Part model, mm, in its own coordinate system. Coordinates: 2 decimals unless noted, no trailing zeros. Loops run counter-clockwise (first coordinate to the right, second up) from the corner with the lowest first, then second, coordinate; pieces in that order, holes last. Notation, with made-up numbers: (-3, -10.75) -> (44, -10.75) arc R9 ccw to (44, 2.25) -> close; hole circle Ø11 at (88, 88). An arc over 180 degrees is marked (long way). Use one line per item in the form item = value. Start each with the question number.
(1) Drill centre lines: L1, parallel to X at y = 5.75, z = 9; L2, parallel to X at y = 13.5, z = 8; L3, parallel to Y at x = 9, z = 22.5. Where is each one in solid material? Low to high. Write a range as [from, to].
(2) Band-saw the part on A-A on z = 23.5. Give the cut face in (x, y).
(3) Pin check, flat tips, straight feed: P1, Ø1.5, axis at y = 4.5, z = 3.5, coming from the +X side; P2, Ø1, axis at y = 5, z = 21.5, coming from the +X side; P3, Ø2, axis at y = 2, z = -3, coming from the +X side. Stop position of each tip, or through.
```python
from build123d import *

# Parameters (mm, degrees)
F0_W         = 15.478125
F0_H         = 15.478125
F1_DEPTH     = 6.35
F2_DEPTH     = 25.4
F2_TAPER     = 10
F3_T1_DEPTH  = 51.3009034407
F3_T3_DEPTH  = 51.3009034407
F3_T5_DEPTH  = 51.3009034407
F3_T7_DEPTH  = 51.3009034407
F3_T9_DEPTH  = 44.45
F3_T11_DEPTH = 0.1267751904
F3_T13_DEPTH = 0.1267751904
F3_S17_W     = 14.1899336178
F3_S17_H     = 14.1899336178
F3_T18_DEPTH = 7.0949668089
F3_S29_W     = 14.1899336177
F3_S29_H     = 14.1899336178
F3_T30_DEPTH = 7.0949668089
F3_S41_W     = 14.1899336177
F3_S41_H     = 14.1899336178
F3_T42_DEPTH = 7.0949668089
F3_S53_W     = 14.1899336178
F3_S53_H     = 14.1899336178
F3_T54_DEPTH = 7.0949668089


# Not quite as in the source:
# - a fillet or chamfer that OpenCascade refuses, or shapes differently, is made with other operations: its cross-section is extruded or revolved along the edge and cut away or added


with BuildPart() as f1:
    # F0 (on Top) → F1 (new body)
    with BuildSketch(Plane.XY):
        with Locations((7.7390625, 7.7390625)):
            Rectangle(F0_W, F0_H)
    extrude(amount=-F1_DEPTH)

    # F0 (on Top) → F2 (join)
    with BuildSketch(Plane.XY):
        with Locations((7.7390625, 7.7390625)):
            Rectangle(F0_W, F0_H)
    extrude(amount=F2_DEPTH, taper=F2_TAPER)

    # F3: fillet of radius 3.81 on 10 edges, made by hand

    # F3_s2 → F3_t1 (cut)
    with BuildSketch(Plane(origin=(5.649698691, 5.649698691, -32.0410334724), x_dir=(0.7071067812, -0.7071067812, 0), z_dir=(-0.1710878697, -0.1710878697, 0.9702875252))):
        with BuildLine():
            ThreePointArc((-2.6531477556, 18.6646706441), (0, 19.7402772951), (2.6531477556, 18.6646706441))
            Line((2.6531477556, 18.6646706441), (0, 21.238986814))
            Line((0, 21.238986814), (-2.6531477556, 18.6646706441))
        make_face()
    extrude(amount=F3_T1_DEPTH, mode=Mode.SUBTRACT)

    # F3_s4 → F3_t3 (cut)
    with BuildSketch(Plane(origin=(-5.1966375782, 5.1966375782, -29.4715962203), x_dir=(0.7071067812, 0.7071067812, 0), z_dir=(0.1710878697, -0.1710878697, 0.9702875252))):
        with BuildLine():
            ThreePointArc((8.2915393919, 8.0451772371), (10.9446871476, 9.1207838881), (13.5978349032, 8.0451772371))
            Line((13.5978349032, 8.0451772371), (10.9446871476, 10.619493407))
            Line((10.9446871476, 10.619493407), (8.2915393919, 8.0451772371))
        make_face()
    extrude(amount=F3_T3_DEPTH, mode=Mode.SUBTRACT)

    # F3_s6 → F3_t5 (cut)
    with BuildSketch(Plane(origin=(5.1966375782, -5.1966375782, -29.4715962203), x_dir=(-0.7071067812, -0.7071067812, 0), z_dir=(-0.1710878697, 0.1710878697, 0.9702875252))):
        with BuildLine():
            ThreePointArc((-8.2915393919, 8.0451772371), (-10.9446871476, 9.1207838881), (-13.5978349032, 8.0451772371))
            Line((-13.5978349032, 8.0451772371), (-10.9446871476, 10.619493407))
            Line((-10.9446871476, 10.619493407), (-8.2915393919, 8.0451772371))
        make_face()
    extrude(amount=F3_T5_DEPTH, mode=Mode.SUBTRACT)

    # F3_s8 → F3_t7 (cut)
    with BuildSketch(Plane(origin=(-4.7435764654, -4.7435764654, -26.9021589682), x_dir=(-0.7071067812, 0.7071067812, 0), z_dir=(0.1710878697, 0.1710878697, 0.9702875252))):
        with BuildLine():
            ThreePointArc((2.6531477556, -2.5743161699), (0, -1.4987095189), (-2.6531477556, -2.5743161699))
            Line((-2.6531477556, -2.5743161699), (0, 0))
            Line((0, 0), (2.6531477556, -2.5743161699))
        make_face()
    extrude(amount=F3_T7_DEPTH, mode=Mode.SUBTRACT)

    # F3_s10 → F3_t9 (cut)
    with BuildSketch(Plane.XY.offset(-15.875)):
        with BuildLine():
            ThreePointArc((0, 3.81), (1.1159231637, 1.1159231637), (3.81, 0))
            Line((3.81, 0), (0, 0))
            Line((0, 0), (0, 3.81))
        make_face()
        with BuildLine():
            ThreePointArc((11.668125, 0), (14.3622018363, 1.1159231637), (15.478125, 3.81))
            Line((15.478125, 3.81), (15.478125, 0))
            Line((15.478125, 0), (11.668125, 0))
        make_face()
    extrude(amount=F3_T9_DEPTH, mode=Mode.SUBTRACT)

    # F3_s12 → F3_t11 (cut)
    with BuildSketch(Plane.XZ.offset(-7.8024500952)):
        with BuildLine():
            ThreePointArc((7.8024500952, 25.4), (10.2514708881, 24.5086293283), (11.5545676342, 22.2515995569))
            Line((11.5545676342, 22.2515995569), (10.99941969, 25.4))
            Line((10.99941969, 25.4), (7.8024500952, 25.4))
        make_face()
        with BuildLine():
            ThreePointArc((3.9235573658, 22.2515995569), (5.2266541119, 24.5086293283), (7.6756749048, 25.4))
            Line((7.6756749048, 25.4), (4.47870531, 25.4))
            Line((4.47870531, 25.4), (3.9235573658, 22.2515995569))
        make_face()
    extrude(amount=F3_T11_DEPTH, mode=Mode.SUBTRACT)

    # F3_s14 → F3_t13 (cut)
    with BuildSketch(Plane.YZ.offset(7.6756749048)):
        with BuildLine():
            ThreePointArc((3.9235573658, 22.2515995569), (5.2266541119, 24.5086293283), (7.6756749048, 25.4))
            Line((7.6756749048, 25.4), (4.47870531, 25.4))
            Line((4.47870531, 25.4), (3.9235573658, 22.2515995569))
        make_face()
        with BuildLine():
            ThreePointArc((11.5545676342, 22.2515995569), (10.2514708881, 24.5086293283), (7.8024500952, 25.4))
            Line((7.8024500952, 25.4), (10.99941969, 25.4))
            Line((10.99941969, 25.4), (11.5545676342, 22.2515995569))
        make_face()
    extrude(amount=F3_T13_DEPTH, mode=Mode.SUBTRACT)


with BuildPart() as f3_tool16:
    # F3_s17 → F3_t18 (new body)
    with BuildSketch(Plane(origin=(11.6595829736, 11.6595829736, 15.951248959), x_dir=(-0.7071067812, 0.7071067812, 0), z_dir=(0.5082206017, 0.5082206017, 0.6952867322))):
        with Locations((0, 7.8454102114)):
            Rectangle(F3_S17_W, F3_S17_H)
    extrude(amount=F3_T18_DEPTH)

    split(bisect_by=Plane.XZ.offset(-7.8024500952), keep=Keep.BOTTOM)

    split(bisect_by=Plane(origin=(-3.1272635948, -3.1272635948, 17.7355931701), x_dir=(0.7071067812, -0.7071067812, 0), z_dir=(-0.1710878697, -0.1710878697, 0.9702875252)), keep=Keep.TOP)

    split(bisect_by=Plane.YZ.offset(7.8024500952), keep=Keep.TOP)

    split(bisect_by=Plane.XY.offset(25.4), keep=Keep.BOTTOM)

    split(bisect_by=Plane(origin=(15.0114024231, 0, 2.6469152655), x_dir=(0, 1, 0), z_dir=(-0.984807753, 0, -0.1736481777)), keep=Keep.TOP)

    split(bisect_by=Plane(origin=(0, 15.0114024231, 2.6469152655), x_dir=(1, 0, 0), z_dir=(0, -0.984807753, -0.1736481777)), keep=Keep.TOP)

    # F3_s25 → F3_t26 (revolve, cut)
    with BuildSketch(Plane(origin=(7.8024500952, 7.8024500952, 21.59), x_dir=(-0.5082206017, -0.5082206017, -0.6952867322), z_dir=(-0.4916419632, -0.4916419632, 0.7187324676))):
        with BuildLine():
            ThreePointArc((0, -3.81), (3.81, 0), (0, 3.81))
            Line((0, 3.81), (0, -3.81))
        make_face()
    revolve(axis=Axis((7.8024500952, 7.8024500952, 21.59), (0.7071067812, -0.7071067812, 0)), mode=Mode.SUBTRACT)


with BuildPart() as f1_1:
    add(f1.part)

    # F3_t15: cut F3_tool16
    add(f3_tool16.part, mode=Mode.SUBTRACT)


with BuildPart() as f3_tool28:
    # F3_s29 → F3_t30 (new body)
    with BuildSketch(Plane(origin=(-7.6617662372, 7.6617662372, 10.4819135463), x_dir=(-0.7071067812, -0.7071067812, 0), z_dir=(-0.5082206017, 0.5082206017, 0.6952867322))):
        with Locations((-10.9446871475, 15.455105973)):
            Rectangle(F3_S29_W, F3_S29_H)
    extrude(amount=F3_T30_DEPTH)

    split(bisect_by=Plane.XZ.offset(-7.8024500952), keep=Keep.BOTTOM)

    split(bisect_by=Plane(origin=(3.5803247075, -3.5803247075, 20.3050304222), x_dir=(0.7071067812, 0.7071067812, 0), z_dir=(0.1710878697, -0.1710878697, 0.9702875252)), keep=Keep.TOP)

    split(bisect_by=Plane.YZ.offset(7.6756749048), keep=Keep.BOTTOM)

    split(bisect_by=Plane.XY.offset(25.4), keep=Keep.BOTTOM)

    split(bisect_by=Plane(origin=(0, 0, 0), x_dir=(0, 1, 0), z_dir=(0.984807753, 0, -0.1736481777)), keep=Keep.TOP)

    split(bisect_by=Plane(origin=(0, 15.0114024231, 2.6469152655), x_dir=(1, 0, 0), z_dir=(0, -0.984807753, -0.1736481777)), keep=Keep.TOP)

    # F3_s37 → F3_t38 (revolve, cut)
    with BuildSketch(Plane(origin=(7.6756749048, 7.8024500952, 21.59), x_dir=(0.5082206017, -0.5082206017, -0.6952867322), z_dir=(0.4916419632, -0.4916419632, 0.7187324676))):
        with BuildLine():
            ThreePointArc((0, -3.81), (3.81, 0), (0, 3.81))
            Line((0, 3.81), (0, -3.81))
        make_face()
    revolve(axis=Axis((7.6756749048, 7.8024500952, 21.59), (0.7071067812, 0.7071067812, 0)), mode=Mode.SUBTRACT)


with BuildPart() as f1_2:
    add(f1_1.part)

    # F3_t27: cut F3_tool28
    add(f3_tool28.part, mode=Mode.SUBTRACT)


with BuildPart() as f3_tool40:
    # F3_s41 → F3_t42 (new body)
    with BuildSketch(Plane(origin=(7.6617662372, -7.6617662372, 10.4819135463), x_dir=(0.7071067812, 0.7071067812, 0), z_dir=(0.5082206017, -0.5082206017, 0.6952867322))):
        with Locations((10.9446871475, 15.455105973)):
            Rectangle(F3_S41_W, F3_S41_H)
    extrude(amount=F3_T42_DEPTH)

    split(bisect_by=Plane.XZ.offset(-7.6756749048), keep=Keep.TOP)

    split(bisect_by=Plane(origin=(-3.5803247075, 3.5803247075, 20.3050304222), x_dir=(-0.7071067812, -0.7071067812, 0), z_dir=(-0.1710878697, 0.1710878697, 0.9702875252)), keep=Keep.TOP)

    split(bisect_by=Plane.YZ.offset(7.8024500952), keep=Keep.TOP)

    split(bisect_by=Plane.XY.offset(25.4), keep=Keep.BOTTOM)

    split(bisect_by=Plane(origin=(15.0114024231, 0, 2.6469152655), x_dir=(0, 1, 0), z_dir=(-0.984807753, 0, -0.1736481777)), keep=Keep.TOP)

    split(bisect_by=Plane(origin=(0, 0, 0), x_dir=(1, 0, 0), z_dir=(0, 0.984807753, -0.1736481777)), keep=Keep.TOP)

    # F3_s49 → F3_t50 (revolve, cut)
    with BuildSketch(Plane(origin=(7.8024500952, 7.6756749048, 21.59), x_dir=(-0.5082206017, 0.5082206017, -0.6952867322), z_dir=(-0.4916419632, 0.4916419632, 0.7187324676))):
        with BuildLine():
            ThreePointArc((0, -3.81), (3.81, 0), (0, 3.81))
            Line((0, 3.81), (0, -3.81))
        make_face()
    revolve(axis=Axis((7.8024500952, 7.6756749048, 21.59), (-0.7071067812, -0.7071067812, 0)), mode=Mode.SUBTRACT)


with BuildPart() as f1_3:
    add(f1_2.part)

    # F3_t39: cut F3_tool40
    add(f3_tool40.part, mode=Mode.SUBTRACT)


with BuildPart() as f3_tool52:
    # F3_s53 → F3_t54 (new body)
    with BuildSketch(Plane(origin=(-3.6639495007, -3.6639495007, 5.0125781335), x_dir=(0.7071067812, -0.7071067812, 0), z_dir=(-0.5082206017, -0.5082206017, 0.6952867322))):
        with Locations((0, 23.0648017346)):
            Rectangle(F3_S53_W, F3_S53_H)
    extrude(amount=F3_T54_DEPTH)

    split(bisect_by=Plane.XZ.offset(-7.6756749048), keep=Keep.TOP)

    split(bisect_by=Plane(origin=(4.0333858203, 4.0333858203, 22.8744676743), x_dir=(-0.7071067812, 0.7071067812, 0), z_dir=(0.1710878697, 0.1710878697, 0.9702875252)), keep=Keep.TOP)

    split(bisect_by=Plane.YZ.offset(7.6756749048), keep=Keep.BOTTOM)

    split(bisect_by=Plane.XY.offset(25.4), keep=Keep.BOTTOM)

    split(bisect_by=Plane(origin=(0, 0, 0), x_dir=(0, 1, 0), z_dir=(0.984807753, 0, -0.1736481777)), keep=Keep.TOP)

    split(bisect_by=Plane(origin=(0, 0, 0), x_dir=(1, 0, 0), z_dir=(0, 0.984807753, -0.1736481777)), keep=Keep.TOP)

    # F3_s61 → F3_t62 (revolve, cut)
    with BuildSketch(Plane(origin=(7.6756749048, 7.6756749048, 21.59), x_dir=(0.5082206017, 0.5082206017, -0.6952867322), z_dir=(0.4916419632, 0.4916419632, 0.7187324676))):
        with BuildLine():
            ThreePointArc((0, -3.81), (3.81, 0), (0, 3.81))
            Line((0, 3.81), (0, -3.81))
        make_face()
    revolve(axis=Axis((7.6756749048, 7.6756749048, 21.59), (-0.7071067812, 0.7071067812, 0)), mode=Mode.SUBTRACT)


with BuildPart() as f1_4:
    add(f1_3.part)

    # F3_t51: cut F3_tool52
    add(f3_tool52.part, mode=Mode.SUBTRACT)


solid = f1_4.part
```
A:
q1.L1 = [1.59, 13.89]
q1.L2 = [3.16, 12.31]
q1.L3 = [4.18, 11.3]
q2.outline = (4.38, 7.68) arc R3.3 ccw to (7.68, 4.38) -> (7.8, 4.38) arc R3.3 ccw to (11.1, 7.68) -> (11.1, 7.8) arc R3.3 ccw to (7.8, 11.1) -> (7.68, 11.1) arc R3.3 ccw to (4.38, 7.8) -> close
q3.P1 = 14.99
q3.P2 = 11.12
q3.P3 = 15.39
